The listing builds one solid part. Answer for the finished solid, in the listing's coordinates (mm). Face numbers are marked on the shaded views. Coordinates: 2 decimals unless noted, no trailing zeros. Order: outer loops, then holes, each group sorted by start corner. A loop starts at its lowest first (then second) coordinate and runs counter-clockwise, first axis right, second up. Notation, with made-up numbers: (-15.75, 19) -> (11.25, 19) arc R30 ccw to (11.25, 57) -> close; hole circle Ø6 at (-23, 68.5). An arc over 180 degrees is marked (long way). Return JSON: item names as keys, results as strings.
```python
from build123d import *

# Parameters (mm, degrees)
F2_W          = 2.54
F2_H          = 91.44
F2_R          = 3.81
F3_DEPTH      = 17.907674907
F3_DEPTH_BACK = 5.081
F4_DEPTH      = 17.907674907
F4_DEPTH_BACK = 5.081


with BuildPart() as f1:
    # F0 (on Top) → F1 (revolve)
    with BuildSketch(Plane.XY):
        Polygon((-15.24, -5.08), (-15.24, 0), (-35.56, 0), (-137.16, -17.91482124), (-137.16, -15.366674907), (-149.86, -15.366674907), (-149.86, -22.986674907), (-137.16, -22.986674907), (-35.60620015, -5.08), align=None)
    revolve(axis=Axis((0, -3.722413492, 0), (0, -1, 0)))

    # F2 (on face) → F3 (cut, two sides)
    with BuildSketch(Plane.XZ.offset(5.08)) as f3_sk:
        Polygon((-114.4246458354, -66.063100075), (-35.2352829134, -20.343100075), (-36.5052829134, -18.1433955494), (-115.6946458354, -63.8633955494), align=None)
        Polygon((-33.9652829134, -22.5428046006), (-35.2352829134, -20.343100075), (-114.4246458354, -66.063100075), (-113.1546458354, -68.2628046006), align=None)
        with Locations((-1.27, 86.40620015)):
            Rectangle(F2_W, F2_H)
        with Locations((1.27, 86.40620015)):
            Rectangle(F2_W, F2_H)
        Polygon((114.4246458354, -66.063100075), (35.2352829134, -20.343100075), (33.9652829134, -22.5428046006), (113.1546458354, -68.2628046006), align=None)
        Polygon((36.5052829134, -18.1433955494), (35.2352829134, -20.343100075), (114.4246458354, -66.063100075), (115.6946458354, -63.8633955494), align=None)
        with Locations((0, 25.4)):
            Circle(F2_R)
        with Locations((-24.1568355139, 7.8490316571)):
            Circle(F2_R)
        with Locations((24.1568355139, 7.8490316571)):
            Circle(F2_R)
        with Locations((14.9297454082, -20.5490316571)):
            Circle(F2_R)
        with Locations((-14.9297454082, -20.5490316571)):
            Circle(F2_R)
    extrude(amount=F3_DEPTH, mode=Mode.SUBTRACT)
    extrude(f3_sk.sketch, amount=-F3_DEPTH_BACK, mode=Mode.SUBTRACT)

    # F2 (on face) → F4 (cut, two sides)
    with BuildSketch(Plane.XZ.offset(5.08)) as f4_sk:
        with BuildLine():
            Line((7.6354261028, 136.9935824331), (15.24, 32.1798677611))
            ThreePointArc((15.24, 32.1798677611), (30.0868740434, 19.041572924), (35.60620015, 0))
            ThreePointArc((35.60620015, 0), (35.5767837041, -1.4470488585), (35.4885829716, -2.8917067269))
            Line((35.4885829716, -2.8917067269), (122.4576355939, -61.8843182428))
            ThreePointArc((122.4576355939, -61.8843182428), (133.4681389299, -31.808760589), (137.20620015, 0))
            ThreePointArc((137.20620015, 0), (99.6824186146, 94.2812641979), (7.6354261028, 136.9935824331))
        make_face()
        with BuildLine():
            ThreePointArc((-35.4885829716, -2.8917067269), (-30.8358738622, 17.803100075), (-15.24, 32.1798677612))
            Line((-15.24, 32.1798677611), (-7.6354261028, 136.9935824331))
            ThreePointArc((-7.6354261028, 136.9935824331), (-118.8240548867, 68.603100075), (-122.4576355939, -61.8843182428))
            Line((-122.4576355939, -61.8843182428), (-35.4885829716, -2.8917067269))
        make_face()
        with BuildLine():
            ThreePointArc((20.2485829716, -29.2881610342), (0, -35.60620015), (-20.2485829716, -29.2881610342))
            Line((-20.2485829716, -29.2881610342), (-114.822209491, -75.1092641903))
            ThreePointArc((-114.822209491, -75.1092641903), (0, -137.20620015), (114.822209491, -75.1092641903))
            Line((114.822209491, -75.1092641903), (20.2485829716, -29.2881610342))
        make_face()
    extrude(amount=F4_DEPTH, mode=Mode.SUBTRACT)
    extrude(f4_sk.sketch, amount=-F4_DEPTH_BACK, mode=Mode.SUBTRACT)


solid = f1.part
```
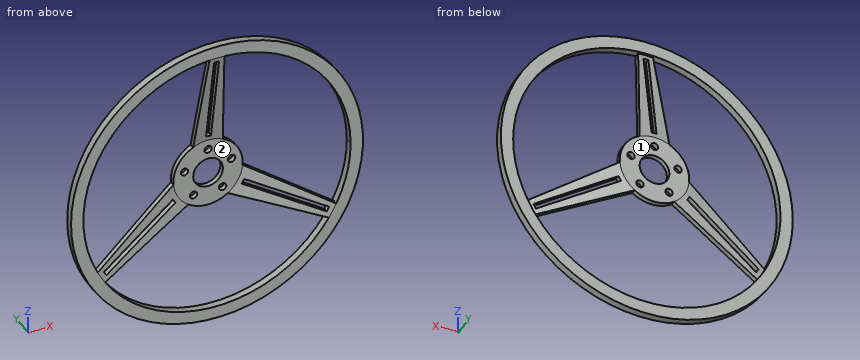
Item 1: Find the intervals of material crossed by probe 1 along Z at (x, y) = (0, -3.9); probe 2 along Z at (x, y) = (14, -20.75); probe 3 along Z at (x, y) = (-44.5, -17), in increasing order.
Answer list:
{"probe 1": "-35.61 to -15.24, 15.24 to 21.59, 29.21 to 40.69", "probe 2": "-149.2 to -136.49, 136.49 to 149.2", "probe 3": "-143.1 to -129.79, 129.79 to 143.1"}
Item 2: The part is cut by section A-A on z = -83.5. Determine the outline of the cut face in (x, y), plus the area to 3 significant figures.
Answer list:
{"outline": "(-124.44, -22.99) -> (-108.87, -22.99) -> (-108.87, -15.37) -> (-124.44, -15.37) -> close; (108.87, -22.99) -> (124.44, -22.99) -> (124.44, -15.37) -> (108.87, -15.37) -> close", "area": "237 mm2"}
Item 3: The part is cut by section B-B on y = -11.5. Determine the outline of the cut face in (x, z).
Answer list:
{"outline": "(-91.97, -41.2) arc R100.78 ccw to (-88.52, -48.17) -> (-63.6, -33.79) arc R72.02 cw to (-67.65, -24.7) -> close; (-85.98, -52.57) arc R100.78 ccw to (-81.67, -59.05) -> (-55.22, -46.23) arc R72.02 cw to (-61.06, -38.19) -> close; (-12.43, 70.94) arc R72.02 cw to (-2.54, 71.97) -> (-2.54, 100.75) arc R100.78 ccw to (-10.3, 100.25) -> close; (2.54, 71.97) arc R72.02 cw to (12.43, 70.94) -> (10.3, 100.25) arc R100.78 ccw to (2.54, 100.75) -> close; (55.22, -46.23) -> (81.67, -59.05) arc R100.78 ccw to (85.98, -52.57) -> (61.06, -38.19) arc R72.02 cw to start; (63.6, -33.79) -> (88.52, -48.17) arc R100.78 ccw to (91.97, -41.2) -> (67.65, -24.7) arc R72.02 cw to start"}
Item 4: The part is cut by section C-C on z = 25.4. Count the separate pieces of the cut face and the enclosed holes in it, plus the area to 3 significant figures.
Answer list:
{"separate pieces": "4", "enclosed holes": "0", "area": "411 mm2"}
Item 5: Flat-ended cylindrical pins translate along their axes: pin 1 (6 mm diameter, centred on y = -5, z = -39.5, fed in from -X); pin 2 (2.5 mm diameter, centred on x = -0.5, y = -3, fed in from +Z); pin 3 (12 mm diameter, centred on x = -24.16, z = 7.85, fed in from -Y). Find the tip coordinate at first contact, or state that the pin passes through.
Answer list:
{"pin 1": "x = -66.25", "pin 2": "z = 40.69", "pin 3": "y = -5.08"}
Item 6: Determine the mould class of the marked faces 1 and 2 for opening direction X: pulls with the +X half, pulls with the -X half, needs draft (parallel to the pull), parting line crosses it, or undercut.
Answer list:
{"face 1": "needs draft", "face 2": "undercut"}
